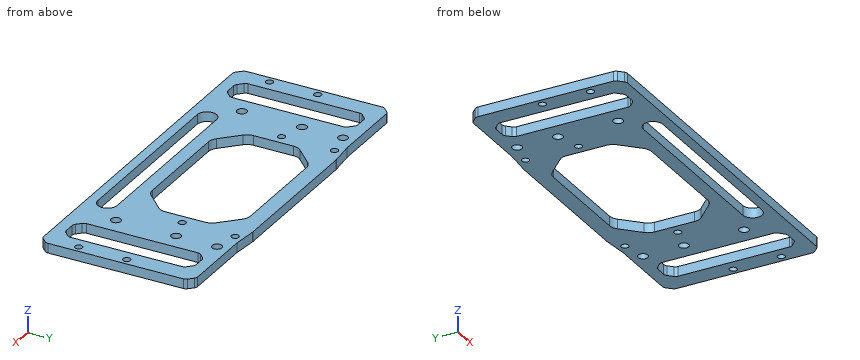
from build123d import *

# Parameters (mm, degrees)
SKETCH_1_W          = 105
SKETCH_1_H          = 52
SKETCH_1_R          = 2.025
SKETCH_1_R_2        = 1.525
SKETCH_1_W_2        = 83
SKETCH_1_H_2        = 1
EXTRUDE_3_DEPTH     = 4
SKETCH_3_W          = 105
SKETCH_3_H          = 12
EXTRUDE_4_DEPTH     = 4
SKETCH_6_W          = 66.47562141
SKETCH_6_H          = 40.771714464
CUT_EXTRUDE_1_DEPTH = 4
CHAMFER_1_SIZE      = 10
FILLET_2_R          = 5
SKETCH_7_W          = 20
SKETCH_7_H          = 64
SKETCH_7_R          = 1.525
EXTRUDE_5_DEPTH     = 4
SKETCH_8_W          = 12
SKETCH_8_H          = 54
CUT_EXTRUDE_2_DEPTH = 10
CUT_EXTRUDE_3_DEPTH = 10
CHAMFER_2_SIZE      = 3
FILLET_3_R          = 2


with BuildPart() as part:
    # 草图1 → 凸台-拉伸3 (new body)
    # profile 1 of 2: a face of its own
    with BuildSketch(Plane.XY):
        Rectangle(SKETCH_1_W, SKETCH_1_H)
        with Locations((-47.5, 4)):
            Circle(SKETCH_1_R, mode=Mode.SUBTRACT)
        with Locations((-47.5, 21)):
            Circle(SKETCH_1_R, mode=Mode.SUBTRACT)
        with Locations((-47.5, -21)):
            Circle(SKETCH_1_R, mode=Mode.SUBTRACT)
        with Locations((47.5, 21)):
            Circle(SKETCH_1_R, mode=Mode.SUBTRACT)
        with Locations((47.5, 4)):
            Circle(SKETCH_1_R, mode=Mode.SUBTRACT)
        with Locations((47.5, -21)):
            Circle(SKETCH_1_R, mode=Mode.SUBTRACT)
        with Locations((-37.5, 23)):
            Circle(SKETCH_1_R_2, mode=Mode.SUBTRACT)
        with Locations((-37.5, 1)):
            Circle(SKETCH_1_R_2, mode=Mode.SUBTRACT)
        with Locations((37.5, 23)):
            Circle(SKETCH_1_R_2, mode=Mode.SUBTRACT)
        with Locations((37.5, 1)):
            Circle(SKETCH_1_R_2, mode=Mode.SUBTRACT)
    # profile 2 of 2: a face of its own
    with BuildSketch(Plane.XY):
        with Locations((0, 26.5)):
            Rectangle(SKETCH_1_W_2, SKETCH_1_H_2)
    extrude(amount=EXTRUDE_3_DEPTH)

    # 草图3 → 凸台-拉伸4 (add)
    with BuildSketch(Plane.XY.offset(4)):
        with Locations((0, -32)):
            Rectangle(SKETCH_3_W, SKETCH_3_H)
        Polygon((-52.5, -26), (-52.5, 26), (-55, 26), (-55, -38), (-52.5, -38), align=None)
        Polygon((52.5, -38), (55, -38), (55, 26), (52.5, 26), (52.5, -26), align=None)
    extrude(amount=-EXTRUDE_4_DEPTH)

    # 草图6 → 切除-拉伸1 (cut)
    with BuildSketch(Plane(origin=(0, 0, 0), x_dir=(-1, 0, 0), z_dir=(0, 0, -1))):
        Rectangle(SKETCH_6_W, SKETCH_6_H)
    extrude(amount=-CUT_EXTRUDE_1_DEPTH, mode=Mode.SUBTRACT)

    # 倒角1
    chamfer_1_edges = [part.edges().sort_by_distance(p)[0] for p in [
        (-33.237810705, -20.385857232, 2),
        (33.237810705, -20.385857232, 2),
        (33.237810705, 20.385857232, 2),
        (-33.237810705, 20.385857232, 2),
    ]]
    chamfer(chamfer_1_edges, length=CHAMFER_1_SIZE)

    # 圆角2
    fillet_2_edges = [part.edges().sort_by_distance(p)[0] for p in [
        (-33.237810705, 10.385857232, 2),
        (-33.237810705, -10.385857232, 2),
        (23.237810705, -20.385857232, 2),
        (-23.237810705, -20.385857232, 2),
        (23.237810705, 20.385857232, 2),
        (-23.237810705, 20.385857232, 2),
        (33.237810705, -10.385857232, 2),
        (33.237810705, 10.385857232, 2),
    ]]
    fillet(fillet_2_edges, radius=FILLET_2_R)

    # 草图7 → 凸台-拉伸5 (add)
    # profile 1 of 2: a face of its own
    with BuildSketch(Plane.XY.offset(4)):
        with Locations((-65, -6)):
            Rectangle(SKETCH_7_W, SKETCH_7_H)
        with Locations((-72, -3)):
            Circle(SKETCH_7_R, mode=Mode.SUBTRACT)
        with Locations((-72, -23)):
            Circle(SKETCH_7_R, mode=Mode.SUBTRACT)
    # profile 2 of 2: a face of its own
    with BuildSketch(Plane.XY.offset(4)):
        with Locations((65, -6)):
            Rectangle(SKETCH_7_W, SKETCH_7_H)
        with Locations((72, -23)):
            Circle(SKETCH_7_R, mode=Mode.SUBTRACT)
        with Locations((72, -3)):
            Circle(SKETCH_7_R, mode=Mode.SUBTRACT)
    extrude(amount=-EXTRUDE_5_DEPTH)

    # 草图8 → 切除-拉伸2 (cut)
    with BuildSketch(Plane.XY.offset(4)):
        with Locations((-61, -6)):
            Rectangle(SKETCH_8_W, SKETCH_8_H)
        with Locations((61, -6)):
            Rectangle(SKETCH_8_W, SKETCH_8_H)
    extrude(amount=-CUT_EXTRUDE_2_DEPTH, mode=Mode.SUBTRACT)

    # 草图9 → 切除-拉伸3 (cut)
    with BuildSketch(Plane.XY.offset(4)):
        Polygon((41.5, 26), (31.5, 27), (41.5, 27), align=None)
        Polygon((-41.5, 27), (-41.5, 26), (-31.5, 27), align=None)
        with BuildLine():
            Line((-37.5, -26), (37.5, -26))
            ThreePointArc((37.5, -26), (41.5, -30), (37.5, -34))
            Line((37.5, -34), (-37.5, -34))
            ThreePointArc((-37.5, -34), (-41.5, -30), (-37.5, -26))
        make_face()
    extrude(amount=-CUT_EXTRUDE_3_DEPTH, mode=Mode.SUBTRACT)

    # 倒角2
    chamfer_2_edges = [part.edges().sort_by_distance(p)[0] for p in [
        (-75, 26, 2),
        (-75, -38, 2),
        (75, -38, 2),
        (75, 26, 2),
        (-67, -33, 2),
        (-67, 21, 2),
        (-55, 21, 2),
        (-55, -33, 2),
        (67, 21, 2),
        (67, -33, 2),
        (55, -33, 2),
        (55, 21, 2),
    ]]
    chamfer(chamfer_2_edges, length=CHAMFER_2_SIZE)

    # 圆角3
    # the kernel refuses this fillet: 2 mm, written as the material it adds along each edge
    with BuildSketch(Plane(origin=(41.5, 26, 0), x_dir=(1, 0, 0), z_dir=(0, 0, 1)), Plane(origin=(-41.5, 26, 0), x_dir=(0.9950371902099869, 0.09950371902102007, 0), z_dir=(0, 0, 1))) as fillet_3_piece_1:
        with BuildLine():
            CenterArc((FILLET_3_R * 0.0498756211208, FILLET_3_R), FILLET_3_R, 264.289406863, 5.710593137)
            Line((-FILLET_3_R * 0.0496280979001, FILLET_3_R * 0.00496280979), (0, 0))
            Line((0, 0), (FILLET_3_R * 0.0498756211209, 0))
        make_face()
    extrude(amount=4)
    with BuildSketch(Plane(origin=(-58, -33, 4), x_dir=(-1, 0, 0), z_dir=(0, 0, -1)), Plane(origin=(-64, -33, 4), x_dir=(-0.7071067811865475, 0.7071067811865475, 0), z_dir=(0, 0, -1)), Plane(origin=(-67, -30, 4), x_dir=(0, 1, 0), z_dir=(0, 0, -1)), Plane(origin=(-55, -30, 4), x_dir=(-0.7071067811865454, -0.7071067811865497, 0), z_dir=(0, 0, -1)), Plane(origin=(55, 18, 4), x_dir=(0.7071067811865475, 0.7071067811865475, 0), z_dir=(0, 0, -1)), Plane(origin=(67, 18, 4), x_dir=(0, -1, 0), z_dir=(0, 0, -1)), Plane(origin=(64, 21, 4), x_dir=(0.7071067811865475, -0.7071067811865475, 0), z_dir=(0, 0, -1)), Plane(origin=(58, 21, 4), x_dir=(1, 0, 0), z_dir=(0, 0, -1))) as fillet_3_piece_2:
        with BuildLine():
            CenterArc((FILLET_3_R * 0.414213562373, FILLET_3_R), FILLET_3_R, 225, 45)
            Line((-FILLET_3_R * 0.292893218813, FILLET_3_R * 0.292893218813), (0, 0))
            Line((0, 0), (FILLET_3_R * 0.414213562373, 0))
        make_face()
    extrude(amount=4)
    with BuildSketch(Plane(origin=(-67, 18, 4), x_dir=(0, -1, 0), z_dir=(0, 0, -1)), Plane(origin=(-55, 18, 4), x_dir=(-0.7071067811865475, 0.7071067811865475, 0), z_dir=(0, 0, -1)), Plane(origin=(-58, 21, 4), x_dir=(-1, 0, 0), z_dir=(0, 0, -1)), Plane(origin=(-64, 21, 4), x_dir=(-0.7071067811865475, -0.7071067811865475, 0), z_dir=(0, 0, -1)), Plane(origin=(64, -33, 4), x_dir=(0.7071067811865475, 0.7071067811865475, 0), z_dir=(0, 0, -1)), Plane(origin=(58, -33, 4), x_dir=(1, 0, 0), z_dir=(0, 0, -1)), Plane(origin=(55, -30, 4), x_dir=(0.7071067811865475, -0.7071067811865475, 0), z_dir=(0, 0, -1)), Plane(origin=(67, -30, 4), x_dir=(0, 1, 0), z_dir=(0, 0, -1))) as fillet_3_piece_3:
        with BuildLine():
            CenterArc((FILLET_3_R * 0.414213562373, -FILLET_3_R), FILLET_3_R, 90, 45)
            Line((-FILLET_3_R * 0.292893218813, -FILLET_3_R * 0.292893218813), (0, 0))
            Line((0, 0), (FILLET_3_R * 0.414213562373, 0))
        make_face()
    extrude(amount=4)
    # the kernel refuses this fillet: 2 mm, written as the material it takes off along each edge
    with BuildSketch(Plane(origin=(-31.5, 27, 4.249378106), x_dir=(1, 0, 0), z_dir=(0, 0, -1)), Plane(origin=(31.5, 27, 4.249378106), x_dir=(0.9950371902099905, -0.0995037190209848, 0), z_dir=(0, 0, -1))) as fillet_3_2_piece_1:
        with BuildLine():
            CenterArc((FILLET_3_R * 0.0498756211209, FILLET_3_R), FILLET_3_R, 264.289406863, 5.710593137)
            Line((-FILLET_3_R * 0.0496280979001, FILLET_3_R * 0.00496280979001), (0, 0))
            Line((0, 0), (FILLET_3_R * 0.0498756211209, 0))
        make_face()
    extrude(amount=4.498756211, mode=Mode.SUBTRACT)
    with BuildSketch(Plane(origin=(-72, -38, 6.071067812), x_dir=(1, 0, 0), z_dir=(0, 0, -1)), Plane(origin=(72, -38, 6.071067812), x_dir=(0.7071067811865475, 0.7071067811865475, 0), z_dir=(0, 0, -1)), Plane(origin=(75, 23, 6.071067812), x_dir=(-0.7071067811865475, 0.7071067811865475, 0), z_dir=(0, 0, -1)), Plane(origin=(75, -35, 6.071067812), x_dir=(0, 1, 0), z_dir=(0, 0, -1)), Plane(origin=(72, 26, 6.071067812), x_dir=(-1, 0, 0), z_dir=(0, 0, -1)), Plane(origin=(-75, -35, 6.071067812), x_dir=(0.7071067811865475, -0.7071067811865475, 0), z_dir=(0, 0, -1))) as fillet_3_2_piece_2:
        with BuildLine():
            CenterArc((FILLET_3_R * 0.414213562373, -FILLET_3_R), FILLET_3_R, 90, 45)
            Line((-FILLET_3_R * 0.292893218813, -FILLET_3_R * 0.292893218813), (0, 0))
            Line((0, 0), (FILLET_3_R * 0.414213562373, 0))
        make_face()
    extrude(amount=8.142135624, mode=Mode.SUBTRACT)
    with BuildSketch(Plane(origin=(-72, 26, 6.071067812), x_dir=(1, 0, 0), z_dir=(0, 0, -1)), Plane(origin=(-75, 23, 6.071067812), x_dir=(0.7071067811865497, 0.7071067811865454, 0), z_dir=(0, 0, -1))) as fillet_3_2_piece_3:
        with BuildLine():
            CenterArc((FILLET_3_R * 0.414213562373, FILLET_3_R), FILLET_3_R, 225, 45)
            Line((-FILLET_3_R * 0.292893218813, FILLET_3_R * 0.292893218813), (0, 0))
            Line((0, 0), (FILLET_3_R * 0.414213562373, 0))
        make_face()
    extrude(amount=8.142135624, mode=Mode.SUBTRACT)


solid = part.part
Work out the finished part from the listing and answer in its coordinate system (mm). Round coordinates to 2 decimals unless told otherwise and drop trailing zeros. Write each loop counter-clockwise with the first axis right and the second up, starting at its lowest first coordinate (ties: lowest second). Pieces come first, ordered by that corner, then holes.
1) A cutting plane is placed at D-D (z = 1.45). Give the number of separate pieces and of enclosed holes in the cut face, plus the area to 3 significant figures.
2) A cutting plane is placed at A-A (y = 4). Give the vertices of the cut face in (x, z) (3 decimals), plus the area to 3 significant figures.
3) Given pin 1 Ø2.5 at (x, y) = (-37.5, 1) entering from -Z, flat-ended and moving along its own axis, determine where the tip first touches the part or whether it passes through.
4) A cutting plane is placed at B-B (x = 23). Give the vertices of the cut face in (y, z).
5) Straight lines are drawn through the part: line 1 (Y direction, x = 6, z = 1.1); line 2 (X direction, y = -25, z = 1.35); line 3 (Y direction, x = -47.5, z = 1.85) (3 decimals). For each, find the intervals that lie inside material, in ascending order.
6) A cutting plane is placed at C-C (y = 14). Give the vertices of the cut face in (x, z), plus the area to 3 significant figures.
Completed:
1. separate pieces: 1
1. enclosed holes: 18
1. area: 5,100 mm2
2. outline: (-75, 0) - (-67, 0) - (-67, 4) - (-75, 4) - close; (-55, 0) - (-49.525, 0) - (-49.525, 4) - (-55, 4) - close; (-45.475, 0) - (-33.238, 0) - (-33.238, 4) - (-45.475, 4) - close; (33.238, 0) - (45.475, 0) - (45.475, 4) - (33.238, 4) - close; (49.525, 0) - (55, 0) - (55, 4) - (49.525, 4) - close; (67, 0) - (75, 0) - (75, 4) - (67, 4) - close
2. area: 206 mm2
3. pin 1: passes through
4. outline: (-38, 0) - (-34, 0) - (-34, 4) - (-38, 4) - close; (-26, 0) - (-20.04, 0) - (-20.04, 4) - (-26, 4) - close; (20.04, 0) - (27, 0) - (27, 4) - (20.04, 4) - close
5. line 1: y = -38 to -34, -26 to -20.39, 20.39 to 27
5. line 2: x = -75 to -67, -55 to 55, 67 to 75
5. line 3: y = -38 to -23.025, -18.975 to 1.975, 6.025 to 18.975, 23.025 to 26
6. outline: (-75, 0) - (-67, 0) - (-67, 4) - (-75, 4) - close; (-55, 0) - (-29.62, 0) - (-29.62, 4) - (-55, 4) - close; (29.62, 0) - (55, 0) - (55, 4) - (29.62, 4) - close; (67, 0) - (75, 0) - (75, 4) - (67, 4) - close
6. area: 267 mm2
